Study the drawing (mm; zero at the part's minimum x, y, z) and answer. Coordinates: 2 decimals unless noted, no trailing zeros. Write each loop counter-clockwise with the first axis right and the second up, starting at its lowest first coordinate (ties: lowest second). Pieces come first, ordered by that corner, then holes. Notation, with made-up numbers: (-21, 83) -> (28, 83) arc R22 cw to (28, 107) -> close; hole circle Ø9 at (4, 87.5). An arc over 180 degrees is marked (long way). Write item = value, one per line. Start each with the question number.
1) Find the intervals of material crossed by line 1 along X through (y, z) = (0.7, 15); line 2 along X through (y, z) = (2.85, 16.75); line 3 along X through (y, z) = (1.9, 8), in increasing order. Write a range as from..to.
2) Section B-B (y = 2.6) is taken. Determine the outline of the cut face in (x, z), plus the area to 3 significant figures.
3) For a pull along Z with two mould halves and no side action, classify the marked faces 1, 2, 3 and 4 as released by +Z, released by -Z, zero draft, split by the parting line, or undercut.
4) Section A-A (x = 15) is taken. Determine the outline of the cut face in (y, z).
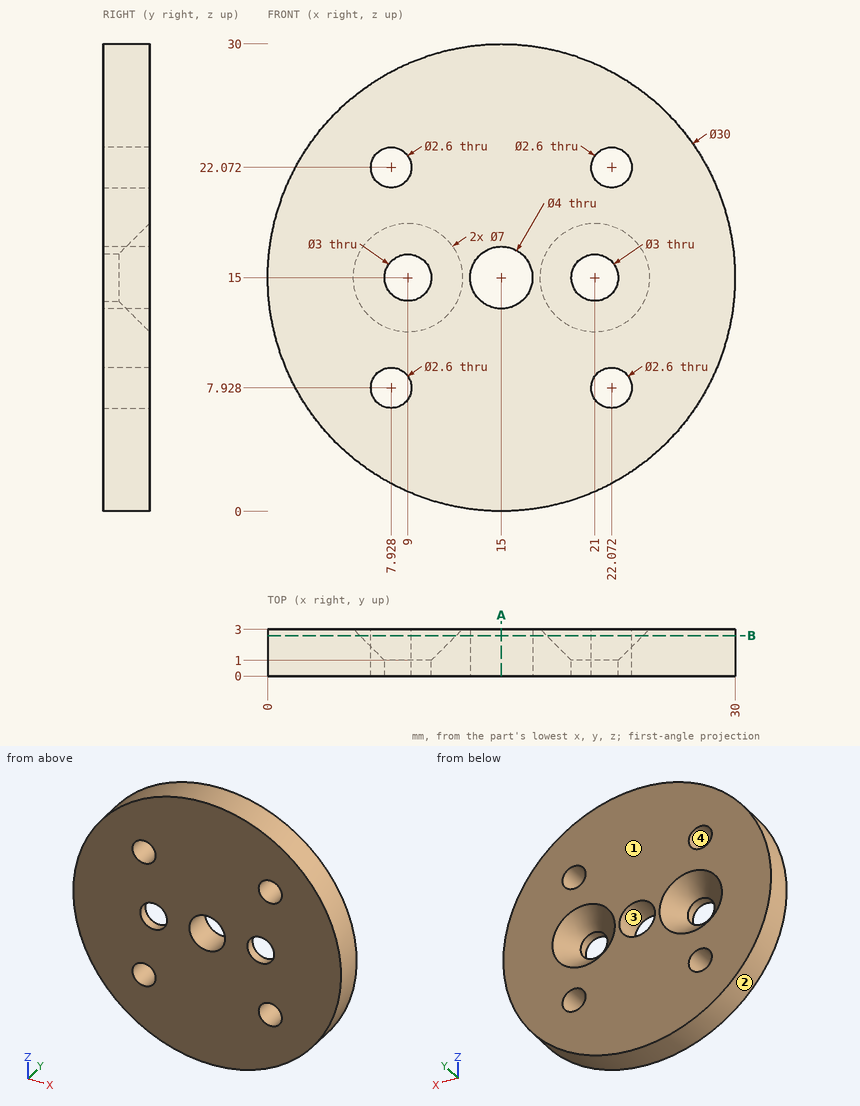
Answer key:
q1.line_1 = 0..7.5, 10.5..13, 17..19.5, 22.5..30
q1.line_2 = 0.1..6.14, 11.86..14.03, 15.97..18.14, 23.86..29.9
q1.line_3 = 1.73..6.63, 9.23..20.77, 23.37..28.27
q2.outline = circle Ø30 at (15, 15); hole circle Ø6.2 at (9, 15); hole circle Ø2.6 at (7.93, 7.93); hole circle Ø2.6 at (7.93, 22.07); hole circle Ø4 at (15, 15); hole circle Ø6.2 at (21, 15); hole circle Ø2.6 at (22.07, 7.93); hole circle Ø2.6 at (22.07, 22.07)
q2.area = 613 mm^2
q3.face_1 = zero draft
q3.face_2 = split by the parting line
q3.face_3 = undercut
q3.face_4 = undercut
q4.outline = (0, 0) -> (3, 0) -> (3, 13) -> (0, 13) -> close; (0, 17) -> (3, 17) -> (3, 30) -> (0, 30) -> close
